Can you work these out from the model? Positions are in its coordinate system, mm. Face numbers are marked on the shaded views. A direction names the side the tool comes from. Round coordinates to 2 decimals unless told otherwise and drop trailing zeros. Order: outer loops, then holes, each group sorted by start corner. A loop starts at its lowest first (then second) coordinate and runs counter-clockwise, first axis right, second up. Notation, with made-up numbers: (-25, 41) -> (-6, 41) arc R11 ccw to (-6, 48) -> close; hole circle Ø9 at (62, -30.75). An arc over 180 degrees is marked (long way). Use a Markdown table: item, result. Add a question column.
Q1. If we section it at A-A on y = 1.45: List the corners of the cut face in (x, z) for me, plus the area to 3 significant figures.
Q2. If we section it at B-B on x = -127.25: List the corners of the cut face in (y, z) for me.
Q3. I need wall thicknesses on line 1 along Z through (x, y) = (-125.75, 3.5); line 2 along X through (y, z) = (1.95, 147); line 3 along Z through (x, y) = (-125, 4.6). Which ranges of each line are inside material? Lowest first, please. Write a range as [from, to].
Q4. We'd pull the mould along Z, two halves only. Please class the marked faces 1, 2 and 3: +Z half, -Z half, draft (parallel to the pull), parting line (faces both ways), or undercut.
Q5. For the marked faces 4 and 5, which set-ups out of +Z, -Z, +X, -X, +Y, -Y let a thin tool reach every point of the face, with its end or its side?
Q6. If we section it at C-C on z = 148.5: List the corners of the cut face in (x, y) for me, plus the area to 3 significant figures.
Q7. I'm going to push flat-ended pins straight in: pin 1 Ø1.5 at (x, y) = (-126.5, 3) entering from +Z; pin 2 Ø0.9 at (x, y) = (-126.5, 2.5) entering from -Z; pin 3 Ø2.5 at (y, z) = (2.5, 154.99) entering from +X. Where does each tip first touch, or does it pass through?
Q8. If we section it at D-D on y = 3.75: List the corners of the cut face in (x, z) for me, plus the area to 3 significant figures.
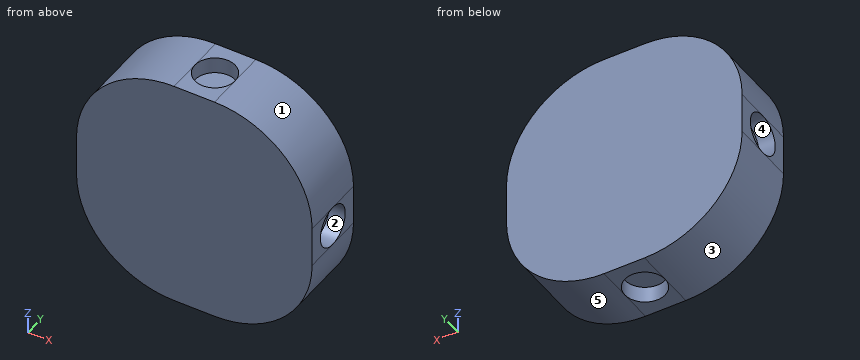
```python
from build123d import *

# Parameters (mm, degrees)
BOSS_EXTRUDE3_DEPTH = 5
SKETCH3_R           = 1.5
CUT_EXTRUDE1_DEPTH  = 1.2
SKETCH4_R           = 1.5
CUT_EXTRUDE2_DEPTH  = 1.2
SKETCH5_R           = 1.5
CUT_EXTRUDE3_DEPTH  = 1.2
SKETCH6_R           = 1.5
CUT_EXTRUDE4_DEPTH  = 1.2


with BuildPart() as part:
    # Sketch1 → Boss-Extrude3 (new body)
    with BuildSketch(Plane(origin=(0, 0, 0), x_dir=(1, 0, 0), z_dir=(0, 1, 0))):
        with BuildLine():
            Line((-128.067602034, -163.739757522), (-125.067602034, -163.739757522))
            ThreePointArc((-125.067602034, -163.739757522), (-119.94107787, -161.616281686), (-117.817602034, -156.489757522))
            Line((-117.817602034, -156.489757522), (-117.817602034, -153.489757522))
            ThreePointArc((-117.817602034, -153.489757522), (-119.94107787, -148.363233359), (-125.067602034, -146.239757522))
            Line((-125.067602034, -146.239757522), (-128.067602034, -146.239757522))
            ThreePointArc((-128.067602034, -146.239757522), (-133.194126197, -148.363233359), (-135.317602034, -153.489757522))
            Line((-135.317602034, -153.489757522), (-135.317602034, -156.489757522))
            ThreePointArc((-135.317602034, -156.489757522), (-133.194126197, -161.616281686), (-128.067602034, -163.739757522))
        make_face()
    extrude(amount=BOSS_EXTRUDE3_DEPTH)

    # Sketch3 → Cut-Extrude1 (cut)
    with BuildSketch(Plane(origin=(0, 0, 146.239757522), x_dir=(-1, 0, 0), z_dir=(0, 0, -1))):
        with Locations((126.567602034, 2.5)):
            Circle(SKETCH3_R)
    extrude(amount=-CUT_EXTRUDE1_DEPTH, mode=Mode.SUBTRACT)

    # Sketch4 → Cut-Extrude2 (cut)
    with BuildSketch(Plane(origin=(-117.817602034, 0, 0), x_dir=(0, 0, -1), z_dir=(1, 0, 0))):
        with Locations((-154.989757522, 2.5)):
            Circle(SKETCH4_R)
    extrude(amount=-CUT_EXTRUDE2_DEPTH, mode=Mode.SUBTRACT)

    # Sketch5 → Cut-Extrude3 (cut)
    with BuildSketch(Plane.ZY.offset(135.317602034)):
        with Locations((154.989757522, 2.5)):
            Circle(SKETCH5_R)
    extrude(amount=-CUT_EXTRUDE3_DEPTH, mode=Mode.SUBTRACT)

    # Sketch6 → Cut-Extrude4 (cut)
    with BuildSketch(Plane.XY.offset(163.739757522)):
        with Locations((-126.567602034, 2.5)):
            Circle(SKETCH6_R)
    extrude(amount=-CUT_EXTRUDE4_DEPTH, mode=Mode.SUBTRACT)


solid = part.part
```
Answer below:
| question | item | result |
|---|---|---|
| 1 | outline | (-135.32, 153.49) arc R7.25 ccw to (-128.07, 146.24) -> (-127.64, 146.24) -> (-127.64, 147.44) -> (-125.5, 147.44) -> (-125.5, 146.24) -> (-125.07, 146.24) arc R7.25 ccw to (-117.82, 153.49) -> (-117.82, 153.92) -> (-119.02, 153.92) -> (-119.02, 156.06) -> (-117.82, 156.06) -> (-117.82, 156.49) arc R7.25 ccw to (-125.07, 163.74) -> (-125.5, 163.74) -> (-125.5, 162.54) -> (-127.64, 162.54) -> (-127.64, 163.74) -> (-128.07, 163.74) arc R7.25 ccw to (-135.32, 156.49) -> (-135.32, 156.06) -> (-134.12, 156.06) -> (-134.12, 153.92) -> (-135.32, 153.92) -> close |
| 1 | area | 251 mm² |
| 2 | outline | (0, 146.24) -> (1.16, 146.24) -> (1.16, 147.44) -> (3.84, 147.44) -> (3.84, 146.24) -> (5, 146.24) -> (5, 163.74) -> (3.84, 163.74) -> (3.84, 162.54) -> (1.16, 162.54) -> (1.16, 163.74) -> (0, 163.74) -> close |
| 3 | line 1 | [147.44, 162.54] |
| 3 | line 2 | [-131.3, -127.96], [-125.17, -121.84] |
| 3 | line 3 | [146.24, 163.74] |
| 4 | face 1 | +Z half |
| 4 | face 2 | undercut |
| 4 | face 3 | -Z half |
| 5 | face 4 | -X |
| 5 | face 5 | -Z, +X, +Y, -Y |
| 6 | outline | (-133.33, 0) -> (-119.81, 0) -> (-119.81, 5) -> (-133.33, 5) -> close |
| 6 | area | 67.6 mm² |
| 7 | pin 1 | z = 162.54 |
| 7 | pin 2 | z = 147.44 |
| 7 | pin 3 | x = -119.02 |
| 8 | outline | (-135.32, 153.49) arc R7.25 ccw to (-128.07, 146.24) -> (-127.4, 146.24) -> (-127.4, 147.44) -> (-125.74, 147.44) -> (-125.74, 146.24) -> (-125.07, 146.24) arc R7.25 ccw to (-117.82, 153.49) -> (-117.82, 154.16) -> (-119.02, 154.16) -> (-119.02, 155.82) -> (-117.82, 155.82) -> (-117.82, 156.49) arc R7.25 ccw to (-125.07, 163.74) -> (-125.74, 163.74) -> (-125.74, 162.54) -> (-127.4, 162.54) -> (-127.4, 163.74) -> (-128.07, 163.74) arc R7.25 ccw to (-135.32, 156.49) -> (-135.32, 155.82) -> (-134.12, 155.82) -> (-134.12, 154.16) -> (-135.32, 154.16) -> close |
| 8 | area | 253 mm² |
